Geometry check sheet. Reference: the model listing, model coordinates, mm. Give positions to 0.01 mm unless a question says otherwise; leave off trailing zeros. Write each loop counter-clockwise with the first axis right and the second up, starting at its lowest first coordinate (ties: lowest second). Pieces come first, ordered by that corner, then holes. Notation, with made-up numbers: (1, 75.25) - (60, 75.25) arc R20 ccw to (60, 109.25) - close; hole circle Ø8 at (-28.5, 80.25). An arc over 180 degrees is marked (long way). Use a Markdown table: item, result.
```python
from build123d import *

# Parameters (mm, degrees)
F0_R     = 3
F0_R_2   = 5
F0_R_3   = 1.75
F0_R_4   = 6
F0_R_5   = 14
F0_R_6   = 29
F0_R_7   = 26
F0_R_8   = 25
F1_DEPTH = 2


with BuildPart() as f1:
    # F0 (on Front) → F1 (new body)
    with BuildSketch(Plane.XZ):
        with BuildLine():
            Line((0, 214), (0, 0))
            Line((0, 0), (410, 0))
            Line((410, 0), (404, 125))
            ThreePointArc((404, 125), (376.308989, 186.308989), (315, 214))
            Line((315, 214), (0, 214))
        make_face()
        with Locations((42, 13)):
            Circle(F0_R, mode=Mode.SUBTRACT)
        with Locations((142, 45)):
            Circle(F0_R_2, mode=Mode.SUBTRACT)
        with Locations((164, 45)):
            Circle(F0_R_2, mode=Mode.SUBTRACT)
        with Locations((186, 45)):
            Circle(F0_R_2, mode=Mode.SUBTRACT)
        with Locations((27, 60)):
            Circle(F0_R_2, mode=Mode.SUBTRACT)
        with Locations((50, 60)):
            Circle(F0_R_2, mode=Mode.SUBTRACT)
        with Locations((73, 60)):
            Circle(F0_R_2, mode=Mode.SUBTRACT)
        with Locations((96, 60)):
            Circle(F0_R_2, mode=Mode.SUBTRACT)
        with Locations((26, 88)):
            Circle(F0_R_3, mode=Mode.SUBTRACT)
        with Locations((74, 88)):
            Circle(F0_R_3, mode=Mode.SUBTRACT)
        with Locations((119, 60)):
            Circle(F0_R_2, mode=Mode.SUBTRACT)
        with Locations((142, 72)):
            Circle(F0_R_4, mode=Mode.SUBTRACT)
        with Locations((164, 72)):
            Circle(F0_R_4, mode=Mode.SUBTRACT)
        with Locations((186, 72)):
            Circle(F0_R_2, mode=Mode.SUBTRACT)
        with Locations((208, 45)):
            Circle(F0_R_2, mode=Mode.SUBTRACT)
        with Locations((230, 45)):
            Circle(F0_R_2, mode=Mode.SUBTRACT)
        with Locations((252, 45)):
            Circle(F0_R_2, mode=Mode.SUBTRACT)
        with Locations((369, 13)):
            Circle(F0_R, mode=Mode.SUBTRACT)
        with Locations((394, 13)):
            Circle(F0_R_4, mode=Mode.SUBTRACT)
        with Locations((208, 72)):
            Circle(F0_R_2, mode=Mode.SUBTRACT)
        with Locations((230, 72)):
            Circle(F0_R_2, mode=Mode.SUBTRACT)
        with Locations((384, 56)):
            Circle(F0_R_5, mode=Mode.SUBTRACT)
        with Locations((50, 112)):
            Circle(F0_R_6, mode=Mode.SUBTRACT)
        with Locations((26, 136)):
            Circle(F0_R_3, mode=Mode.SUBTRACT)
        with Locations((74, 136)):
            Circle(F0_R_3, mode=Mode.SUBTRACT)
        with Locations((115, 112)):
            Circle(F0_R_7, mode=Mode.SUBTRACT)
        with Locations((180, 112)):
            Circle(F0_R_7, mode=Mode.SUBTRACT)
        with Locations((50, 175)):
            Circle(F0_R_7, mode=Mode.SUBTRACT)
        with Locations((8, 203)):
            Circle(F0_R, mode=Mode.SUBTRACT)
        with Locations((115, 175)):
            Circle(F0_R_7, mode=Mode.SUBTRACT)
        with Locations((180, 175)):
            Circle(F0_R_7, mode=Mode.SUBTRACT)
        with Locations((243, 112)):
            Circle(F0_R_7, mode=Mode.SUBTRACT)
        with Locations((370, 108)):
            Circle(F0_R_8, mode=Mode.SUBTRACT)
        with Locations((243, 175)):
            Circle(F0_R_7, mode=Mode.SUBTRACT)
    extrude(amount=F1_DEPTH)


solid = f1.part
```
1) Depth check by flat-ended pin: P1, Ø8, axis at x = 186, z = 72, coming from the +Y side. Enter the tip coordinate at first touch or a pass-through.
Working result:
| item | result |
|---|---|
| P1 | passes through |
2) Mould release check, pull along X, two halves, no side actions. Record for faces 1 (the cylindrical face through (234.77, -0.99, 46.5)), 2 (the flat face through (202, 0, 85)), 3 (the cylindrical face through (267, -1, 165)): pulls with the +X half, pulls with the -X half, needs draft (parallel to the pull), parting line crosses it, or undercut.
Working result:
| item | result |
|---|---|
| face 1 | undercut |
| face 2 | needs draft |
| face 3 | undercut |
3) Section check A-A on x = 96. Record the boundary of the cut face in (y, z).
Working result:
| item | result |
|---|---|
| outline | (-2, 0) - (0, 0) - (0, 55) - (-2, 55) - close; (-2, 65) - (0, 65) - (0, 94.25) - (-2, 94.25) - close; (-2, 129.75) - (0, 129.75) - (0, 157.25) - (-2, 157.25) - close; (-2, 192.75) - (0, 192.75) - (0, 214) - (-2, 214) - close |
4) Material ranges on L1, parallel to Z at x = 113.5, y = -0.3; L2, parallel to X at y = -1.4, z = 91; L3, parallel to Z at x = 201.5, y = -0.45, recorded low to high. Write a range as from..to.
Working result:
| item | result |
|---|---|
| L1 | z = 0..86.04, 137.96..149.04, 200.96..214 |
| L2 | x = 0..30, 70..99.67, 130.33..164.67, 195.33..227.67, 258.33..351.67, 388.33..405.63 |
| L3 | z = 0..97.38, 126.62..160.38, 189.62..214 |
5) Section check B-B on z = 112. Record the boundary of the cut face in (x, y).
Working result:
| item | result |
|---|---|
| outline | (0, -2) - (21, -2) - (21, 0) - (0, 0) - close; (79, -2) - (89, -2) - (89, 0) - (79, 0) - close; (141, -2) - (154, -2) - (154, 0) - (141, 0) - close; (206, -2) - (217, -2) - (217, 0) - (206, 0) - close; (269, -2) - (345.32, -2) - (345.32, 0) - (269, 0) - close; (394.68, -2) - (404.62, -2) - (404.62, 0) - (394.68, 0) - close |
6) Section check C-C on y = -1.15. Count the separate pieces of the cut face and the enclosed holes in it, then the cut area to 3 significant figures.
Working result:
| item | result |
|---|---|
| separate pieces | 1 |
| enclosed holes | 34 |
| area | 63,300 mm² |
